Autodesk Inventor part; units mm, degrees
ref_plane "YZ Plane" through (0, 0, 0) normal (1, 0, 0) x (0, 1, 0)
ref_plane "XZ Plane" through (0, 0, 0) normal (0, 1, 0) x (-1, 0, 0)
ref_plane "XY Plane" through (0, 0, 0) normal (0, 0, 1) x (1, 0, 0)
sketch "base_sketch" plane through (0, 0, 0) normal (0, 0, 1) x (1, 0, 0)
  line L0 (0, 0) -> (50.8, 0)
  line L1 (50.8, 0) -> (50.8, 30.48)
  line L2 (50.8, 30.48) -> (0, 30.48)
  line L3 (0, 30.48) -> (0, 0)
  dimension "d0" = 50.8
  dimension "d1" = 30.48
extrude "base_extrusion" add sketch "base_sketch" along normal blind 5.08
sketch "moon_sketch" plane through (0, 0, 5.08) normal (0, 0, 1) x (1, 0, 0)
  line L0 (0, 30.48) -> (0, 0)
  line L1 (0, 15.24) -> (25.4, 15.24) construction
  line L2 (25.4, 15.24) -> (50.8, 15.24) construction
  line L3 (25.4, 30.48) -> (25.4, 15.24)
  line L4 (0, 0) -> (50.8, 0)
  line L5 (25.4, 0) -> (25.4, 15.24)
  line L6 (50.8, 30.48) -> (0, 30.48)
  line L7 (25.4, 30.48) -> (43.18, 30.48)
  line L8 (43.18, 30.48) -> (43.18, 25.4)
  line L9 (43.18, 25.4) -> (40.894, 25.4)
  line L10 (40.894, 25.4) -> (40.894, 5.08)
  line L11 (40.894, 5.08) -> (43.18, 5.08)
  line L12 (43.18, 5.08) -> (43.18, 0)
  dimension "d4" = 17.78
  dimension "d5" = 5.08
  dimension "d6" = 2.286
revolve "moon_revolution" add sketch "moon_sketch" angle 180 about axis through (25.4, 30.48, 5.08) along (0, -1, 0) contours L6 L8 L9 L10 L11 L12 L4 L5 L3
sketch "cutout_sketch" plane through (0, 0, 0) normal (0, -1, 0) x (1, 0, 0)
  line L0 (43.18, 5.08) -> (7.62, 5.08)
  line L1 (42.8625, 5.08) -> (46.0375, 5.08)
  arc A0 (40.894, 5.08) -> (9.906, 5.08) centre (25.4, 5.08) ccw
  circle A1 centre (25.4, 5.08) radius 10.414
  line L2 (35.814, 5.08) -> (14.986, 5.08)
  point P0 (0, 0)
  point P1 (53.594, 5.08)
  point P2 (-2.794, 5.08)
  dimension "d16" = 5.08
extrude "cutout_extrusion" cut sketch "cutout_sketch" against normal up to next contours L0 A1 picked at (24.9454, 10.8279)
sketch "peg_sketch" plane through (0, 0, 0) normal (0, 0, -1) x (-1, 0, 0)
  line L0 (-50.8, 17.78) -> (-48.26, 17.78)
  line L1 (-48.26, 17.78) -> (-48.26, 12.7)
  line L2 (-48.26, 12.7) -> (-50.8, 12.7)
  line L3 (-50.8, 0) -> (-50.8, 30.48)
  line L4 (-50.8, 0) -> (-50.8, 12.7) construction
  line L5 (-50.8, 30.48) -> (-50.8, 17.78) construction
  line L6 (-50.8, 17.78) -> (-50.8, 12.7)
  line L7 (-2.54, 17.78) -> (0, 17.78)
  line L8 (0, 17.78) -> (0, 12.7)
  line L9 (0, 12.7) -> (-2.54, 12.7)
  line L10 (-2.54, 12.7) -> (-2.54, 17.78)
  line L11 (0, 30.48) -> (0, 17.78) construction
  line L12 (0, 12.7) -> (0, 0) construction
  line L13 (0, 30.48) -> (0, 0) construction
  dimension "d19" = 5.08
  dimension "d20" = 2.54
  dimension "d21" = 5.08
  dimension "d22" = 2.54
extrude "peg_extrusion" add sketch "peg_sketch" along normal blind 5.08
sketch "rivet_groove_sketch" plane through (0, 0, 0) normal (0, -1, 0) x (1, 0, 0)
  line L0 (20.32, 1.27) -> (30.48, 1.27)
  line L1 (30.48, 1.27) -> (30.48, 0)
  line L2 (30.48, 0) -> (20.32, 0)
  line L3 (20.32, 0) -> (20.32, 1.27)
  line L4 (50.8, 0) -> (30.48, 0) construction
  line L5 (0, 0) -> (20.32, 0) construction
  line L6 (50.8, 0) -> (50.8, 5.08)
  line L7 (0, 0) -> (50.8, 0)
  dimension "d25" = 10.16
  dimension "d26" = 1.27
extrude "rivet_groove_extrusion" cut sketch "rivet_groove_sketch" against normal up to next
equation "\"d0\" = hm_base_length"
equation "\"d1\" = hm_base_width"
equation "\"d2\" = hm_base_height"
equation "\"d4\" = hm_moon_flange_radius"
equation "\"d5\" = hm_moon_flange_width"
equation "\"d6\" = hm_moon_channel_offset"
equation "\"d16\" = hm_moon_thickness"
equation "\"d19\" = hm_peg_length"
equation "\"d20\" = hm_peg_width"
equation "\"d21\" = hm_peg_length"
equation "\"d22\" = hm_peg_width"
equation "\"d23\" = hm_peg_height"
equation "\"d25\" = hm_rivet_groove_width"
equation "\"d26\" = hm_rivet_groove_height"
equation "\"d27\" = hm_peg_height"
equation "\"hm_base_width\" = 30.48"
equation "\"hm_base_length\" = 50.8"
equation "\"hm_moon_flange_radius\" = 17.78"
equation "\"hm_moon_channel_offset\" = 2.286"
equation "\"hm_moon_flange_width\" = 5.08"
equation "\"hm_moon_thickness\" = 5.08"
equation "\"hm_peg_width\" = 2.54"
equation "\"hm_peg_length\" = 5.08"
equation "\"hm_base_height\" = 5.08"
equation "\"hm_peg_height\" = 5.08"
equation "\"hm_rivet_groove_width\" = 10.16"
equation "\"hm_rivet_groove_height\" = 1.27"
properties part number "half_moon(hm)" material "ABS Plastic"
Model file for the job. Use its own axes, mm. A direction names the side the tool comes from. Give positions to 0.01 mm unless a question says otherwise; leave off trailing zeros. Loops run counter-clockwise (first coordinate to the right, second up) from the corner with the lowest first, then second, coordinate; pieces in that order, holes last. Notation, with made-up numbers: M 39.25,63 L 80.25,63 A11 ccw 80.25,74 Z; hole C 14,76.5 d3. An arc over 180 degrees is marked long. Use one line per item in the form item = value.
Item 1: Slice it at B-B on y = 8.5. List the corners of the cut face in (x, z).
Filled in:
outline = M 0,0 L 20.32,0 L 20.32,1.27 L 30.48,1.27 L 30.48,0 L 50.8,0 L 50.8,5.08 L 40.89,5.08 A15.49 ccw 9.91,5.08 L 0,5.08 Z; hole M 14.99,5.08 L 35.81,5.08 A10.41 ccw Z
Item 2: Flat gauge pins, fed straight in: pin 1 Ø1.3 at (x, z) = (1.5, -4) entering from -Y; pin 2 Ø8 at (x, y) = (47.5, 17.5) entering from +Z; pin 3 Ø1.5 at (x, y) = (43.5, 22) entering from -Z. Where does each tip first touch, or does it go through?
Filled in:
pin_1 = 12.7
pin_2 = 5.08
pin_3 = 0
Item 3: Slice it at A-A on z = -2.75. List the corners of the cut face in (x, y).
Filled in:
outline = M 0,12.7 L 2.54,12.7 L 2.54,17.78 L 0,17.78 Z; M 48.26,12.7 L 50.8,12.7 L 50.8,17.78 L 48.26,17.78 Z
Item 4: Which spindle directions (+Z, -Z, +X, -X, +Y, -Y) get a long thin tool onto all of the face, cutting with end or side? Do faces 1 (the flat face through (50, 12.7, -3)), 2 (the flat face through (26, 15, 5.08)), 3 (the flat face through (5, 15, 5.08)), 4 (the flat face through (50, 17.78, -3)). Say none if no direction does.
Filled in:
face_1 = -Z, +X, -X, -Y
face_2 = +Y, -Y
face_3 = +Z, -X
face_4 = -Z, +X, -X, +Y
Item 5: Two-plate mould, pull along X, no slides. Class faces 5 (the flat face through (50.8, 15, 2)), 6 (the flat face through (25, 15, 1.27)), 7 (the cylindrical face through (25.63, 15.03, 15.49)), 8 (the flat face through (26, 30.48, 4)): released by +X, released by -X, zero draft, split by the parting line, or undercut.
Filled in:
face_5 = released by +X
face_6 = undercut
face_7 = undercut
face_8 = zero draft
Item 6: Slice it at C-C on x = 25.4. List the corners of the cut face in (y, z).
Filled in:
outline = M 0,1.27 L 30.48,1.27 L 30.48,5.08 L 0,5.08 Z; M 0,15.49 L 30.48,15.49 L 30.48,22.86 L 25.4,22.86 L 25.4,20.57 L 5.08,20.57 L 5.08,22.86 L 0,22.86 Z
Item 7: Drill centre lines: L1, parallel to Y at x = 9.5, z = 9.5; L2, parallel to X at y = 15.5, z = -2; L3, parallel to Z at x = 9, y = 5.5. Where is each one in solid material? Low to high.
Filled in:
L1 = 0 to 5.08, 25.4 to 30.48
L2 = 0 to 2.54, 48.26 to 50.8
L3 = 0 to 5.08
Item 8: Slice it at D-D on y = 2. List the corners of the cut face in (x, z), and give its area (3 significant figures).
Filled in:
outline = M 0,0 L 20.32,0 L 20.32,1.27 L 30.48,1.27 L 30.48,0 L 50.8,0 L 50.8,5.08 L 43.18,5.08 A17.78 ccw 7.62,5.08 L 0,5.08 Z; hole M 14.99,5.08 L 35.81,5.08 A10.41 ccw Z
area = 571 mm^2
